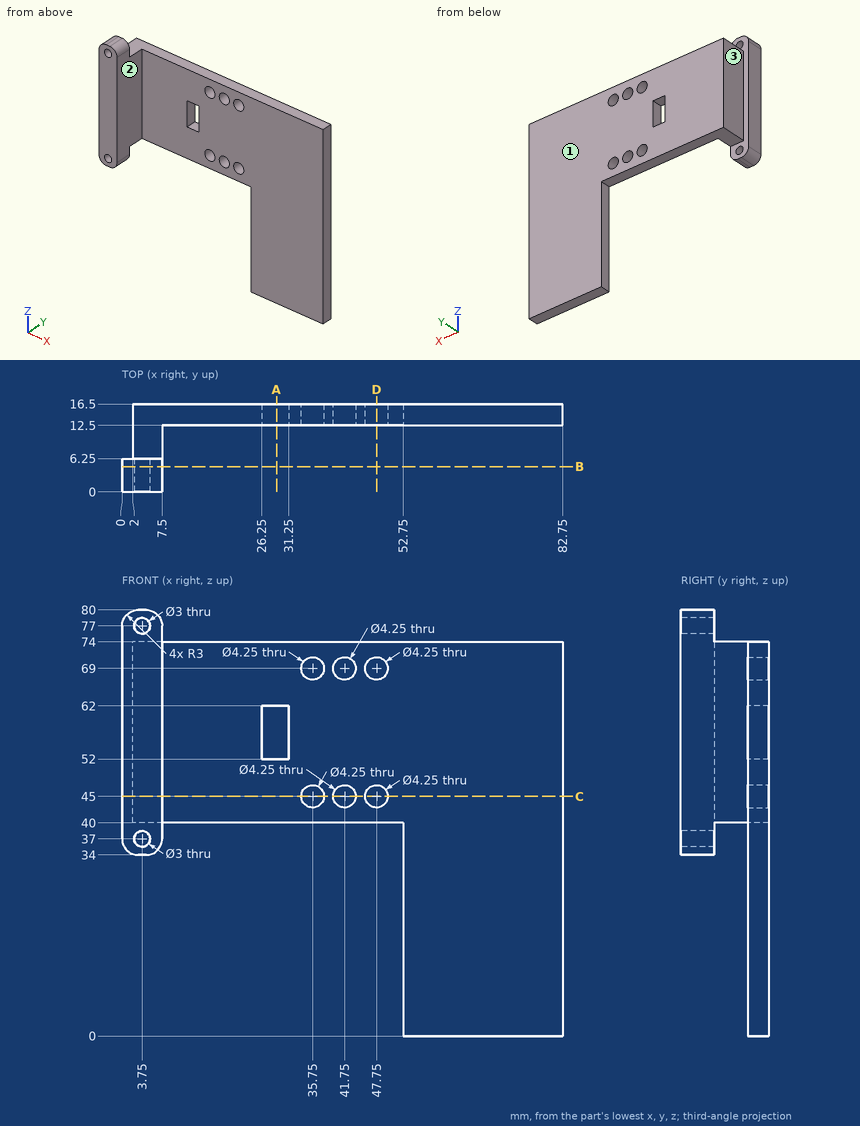
Part print with two shaded views. Sizes in mm from the minimum x, y, z corner. A direction names the side the tool comes from. Round coordinates to 2 decimals unless told otherwise and drop trailing zeros. Order: outer loops, then holes, each group sorted by start corner. A loop starts at its lowest first (then second) coordinate and runs counter-clockwise, first axis right, second up. Notation, with made-up numbers: (-3.5, 18) -> (5.5, 18) arc R12 cw to (5.5, 35) -> close; hole circle Ø2 at (-1.75, 35.5). An arc over 180 degrees is marked (long way). Use one line per item in the form item = value.
Item 1: Cut at B-B, the plane y = 4.75. Write the cut outline in (x, z), and give its area (3 significant figures).
Returned:
outline = (0, 37) arc R3 ccw to (3, 34) -> (4.5, 34) arc R3 ccw to (7.5, 37) -> (7.5, 77) arc R3 ccw to (4.5, 80) -> (3, 80) arc R3 ccw to (0, 77) -> close; hole circle Ø3 at (3.75, 37); hole circle Ø3 at (3.75, 77)
area = 323 mm^2
Item 2: Tool access for the marked faces 1, 2 and 3: list every direction of +Z, -Z, +X, -X, +Y, -Y with a clear straight run to the whole face (end or side of a thin tool).
Returned:
face_1 = +Z, -Z, +X, -X, +Y
face_2 = +Z, -Z, +X, -Y
face_3 = +Z, -Z, -X, +Y
Item 3: Drill centre lines: line 1 (Z direction, x = 41.75, y = 13.8) (3 decimals); line 2 (X direction, y = 14.9, z = 45) (3 decimals); line 3 (X direction, y = 8.75, z = 72). Where is each one in solid material? Low to high.
Returned:
line_1 = 40 to 42.875, 47.125 to 66.875, 71.125 to 74
line_2 = 2 to 33.625, 37.875 to 39.625, 43.875 to 45.625, 49.875 to 82.75
line_3 = 2 to 7.5
Item 4: Cut at A-A, the plane x = 29. Write the cut outline in (y, z), and give its area (3 significant figures).
Returned:
outline = (12.5, 40) -> (16.5, 40) -> (16.5, 52) -> (12.5, 52) -> close; (12.5, 62) -> (16.5, 62) -> (16.5, 74) -> (12.5, 74) -> close
area = 96.0 mm^2
Item 5: Cut at D-D, the plane x = 47.75. Write the cut outline in (y, z) (3 decimals), and give its area (3 significant figures).
Returned:
outline = (12.5, 40) -> (16.5, 40) -> (16.5, 42.875) -> (12.5, 42.875) -> close; (12.5, 47.125) -> (16.5, 47.125) -> (16.5, 66.875) -> (12.5, 66.875) -> close; (12.5, 71.125) -> (16.5, 71.125) -> (16.5, 74) -> (12.5, 74) -> close
area = 102 mm^2
Item 6: Cut at C-C, the plane z = 45. Write the cut outline in (x, y) (3 decimals).
Returned:
outline = (0, 0) -> (7.5, 0) -> (7.5, 12.5) -> (33.625, 12.5) -> (33.625, 16.5) -> (2, 16.5) -> (2, 6.25) -> (0, 6.25) -> close; (37.875, 12.5) -> (39.625, 12.5) -> (39.625, 16.5) -> (37.875, 16.5) -> close; (43.875, 12.5) -> (45.625, 12.5) -> (45.625, 16.5) -> (43.875, 16.5) -> close; (49.875, 12.5) -> (82.75, 12.5) -> (82.75, 16.5) -> (49.875, 16.5) -> close
Item 7: Flat gauge pins, fed straight in: pin 1 Ø3 at (y, z) = (7, 35.5) entering from -X; pin 2 Ø1.2 at (y, z) = (14, 57.5) entering from -X; pin 3 Ø3 at (x, y) = (27.5, 14) entering from -Z. Where does each tip first touch, or does it go through?
Returned:
pin_1 = 0.01
pin_2 = 2
pin_3 = 40
